```python
from build123d import *

# Parameters (mm, degrees)
SKETCH_1_R      = 1.5
SKETCH_1_R_2    = 4
EXTRUDE_1_DEPTH = 3
FILLET_2_R      = 3


with BuildPart() as part:
    # 草图1 → 凸台-拉伸1 (new body)
    with BuildSketch(Plane(origin=(0, 0, 0), x_dir=(1, 0, 0), z_dir=(0, 1, 0))):
        Polygon((25, 17.5), (25, -27.5), (-25, -27.5), (-25, 17.5), (-25, 62.5), (25, 62.5), align=None)
        with Locations(Location((0, 57, 0), (0, 0, 270))):
            Circle(SKETCH_1_R, mode=Mode.SUBTRACT)
        with Locations(Location((10.5, 32.5, 0), (0, 0, 270))):
            Circle(SKETCH_1_R, mode=Mode.SUBTRACT)
        with Locations(Location((21, 57, 0), (0, 0, 270))):
            Circle(SKETCH_1_R, mode=Mode.SUBTRACT)
        with Locations(Location((0, -10, 0), (0, 0, 270))):
            Circle(SKETCH_1_R_2, mode=Mode.SUBTRACT)
        with Locations(Location((0, -3, 0), (0, 0, 270))):
            Circle(SKETCH_1_R, mode=Mode.SUBTRACT)
        with Locations(Location((-18.5, -10, 0), (0, 0, 270))):
            Circle(SKETCH_1_R, mode=Mode.SUBTRACT)
        with Locations(Location((18.5, -10, 0), (0, 0, 270))):
            Circle(SKETCH_1_R, mode=Mode.SUBTRACT)
        with Locations(Location((7, -10, 0), (0, 0, 270))):
            Circle(SKETCH_1_R, mode=Mode.SUBTRACT)
        with Locations(Location((0, -17, 0), (0, 0, 270))):
            Circle(SKETCH_1_R, mode=Mode.SUBTRACT)
        with Locations(Location((-7, -10, 0), (0, 0, 270))):
            Circle(SKETCH_1_R, mode=Mode.SUBTRACT)
    extrude(amount=EXTRUDE_1_DEPTH)

    # 圆角2
    fillet_2_edges = [part.edges().sort_by_distance(p)[0] for p in [
        (25, 1.5, 27.5),
        (-25, 1.5, 27.5),
        (-25, 1.5, -62.5),
        (25, 1.5, -62.5),
    ]]
    fillet(fillet_2_edges, radius=FILLET_2_R)


solid = part.part
```
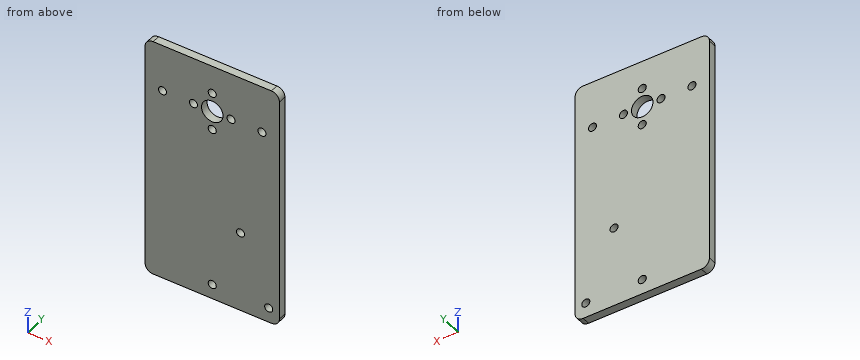
Verification items for the finished model (mm, model axes). Coordinates: 2 decimals unless noted, no trailing zeros. Loops run counter-clockwise (first coordinate to the right, second up) from the corner with the lowest first, then second, coordinate; pieces in that order, holes last. Notation, with made-up numbers: (14.25, -1.5) -> (28.25, -1.5) arc R25 cw to (28.25, 14.5) -> close; hole circle Ø6 at (23, 76.5). An arc over 180 degrees is marked (long way). Answer in a Markdown table with one row per item. Add a question column.
1. Section check C-C, the plane z = -57. Enter the section's corners in (x, y), then the cut area to 3 significant figures.
2. Depth check by flat-ended pin: P1, Ø6, axis at x = -18, z = -38.5, coming from the -Y side. Enter the tip coordinate at first touch or a pass-through.
3. Section check B-B, the plane x = 0. Enter the section's corners in (y, z).
4. Section check A-A, the plane z = 3. Enter the section's corners in (x, y), then the cut area to 3 significant figures.
5. Material ranges on probe 1 along X at (y, z) = (2.35, 10); probe 2 along X at (y, z) = (1.05, -57); probe 3 along X at (y, z) = (1.7, 3), recorded low to high. Write a range as [from, to].
6. Section check D-D, the plane y = 0.7. Give the number of separate pieces and of enclosed holes in the cut face, then the cut area to 3 significant figures.
Derived:
| question | item | result |
|---|---|---|
| 1 | outline | (-25, 0) -> (-1.5, 0) -> (-1.5, 3) -> (-25, 3) -> close; (1.5, 0) -> (19.5, 0) -> (19.5, 3) -> (1.5, 3) -> close; (22.5, 0) -> (25, 0) -> (25, 3) -> (22.5, 3) -> close |
| 1 | area | 132 mm² |
| 2 | P1 | stops at y = 0 |
| 3 | outline | (0, -62.5) -> (3, -62.5) -> (3, -58.5) -> (0, -58.5) -> close; (0, -55.5) -> (3, -55.5) -> (3, 1.5) -> (0, 1.5) -> close; (0, 4.5) -> (3, 4.5) -> (3, 6) -> (0, 6) -> close; (0, 14) -> (3, 14) -> (3, 15.5) -> (0, 15.5) -> close; (0, 18.5) -> (3, 18.5) -> (3, 27.5) -> (0, 27.5) -> close |
| 4 | outline | (-25, 0) -> (-1.5, 0) -> (-1.5, 3) -> (-25, 3) -> close; (1.5, 0) -> (25, 0) -> (25, 3) -> (1.5, 3) -> close |
| 4 | area | 141 mm² |
| 5 | probe 1 | x = [-25, -20], [-17, -8.5], [-5.5, -4], [4, 5.5], [8.5, 17], [20, 25] |
| 5 | probe 2 | x = [-25, -1.5], [1.5, 19.5], [22.5, 25] |
| 5 | probe 3 | x = [-25, -1.5], [1.5, 25] |
| 6 | separate pieces | 1 |
| 6 | enclosed holes | 10 |
| 6 | area | 4,380 mm² |
